Design review of the part shown in the three views and the two pictorial views. Dimensions are in mm from the part's minimum x, y and z. A direction names the side the tool comes from. Round coordinates to 2 decimals unless told otherwise and drop trailing zeros. Order: outer loops, then holes, each group sorted by start corner. A loop starts at its lowest first (then second) coordinate and runs counter-clockwise, first axis right, second up.
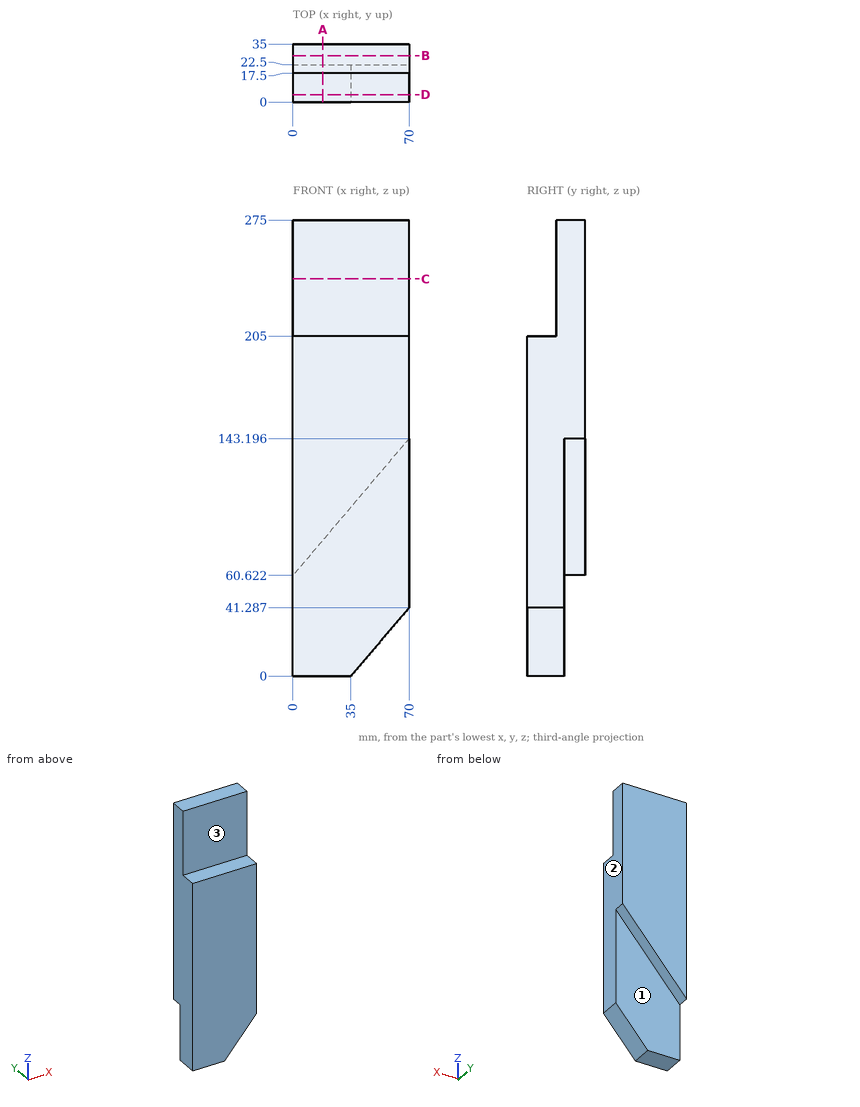
1) To check wall thickness, follow line 1 along Y through (x, z) = (4, 218); line 2 along Y through (x, z) = (9, 61); line 3 along Z through (x, y) = (20, 7). State the ranges of each line that lie inside material, in increasing order.
Results:
line 1: y = 17.5 to 35
line 2: y = 0 to 22.5
line 3: z = 0 to 205
2) Take a section at A-A on x = 18. Give the boundary of the cut face in (y, z) (1 decimal), plus the area to 3 significant figures.
Results:
outline: (0, 0) - (22.5, 0) - (22.5, 81.9) - (35, 81.9) - (35, 275) - (17.5, 275) - (17.5, 205) - (0, 205) - close
area: 7,380 mm2
3) Take a section at C-C on z = 239.5. Give the boundary of the cut face in (x, y), plus the area to 4 significant figures.
Results:
outline: (0, 17.5) - (70, 17.5) - (70, 35) - (0, 35) - close
area: 1,225 mm2
4) Clearance check with flat-ended pins moving along their axes: P1, Ø19, axis at x = 39.5, y = 6, coming from the +Z side; P2, Ø21, axis at x = 17.5, z = 43, coming from the +Y side; P3, Ø4, axis at x = 35, y = 28, coming from the -Z side. State where each tip first meets the part, or that it passes through.
Results:
P1: stops at z = 205
P2: stops at y = 22.5
P3: stops at z = 99.55
5) Take a section at D-D on y = 4.5. Give the boundary of the cut face in (x, z), plus the area to 3 significant figures.
Results:
outline: (0, 0) - (35, 0) - (70, 41.29) - (70, 205) - (0, 205) - close
area: 13,600 mm2
6) Take a section at B-B on y = 28. Give the boundary of the cut face in (x, z).
Results:
outline: (0, 60.62) - (70, 143.2) - (70, 275) - (0, 275) - close
7) For the marked faces 1, 2 and 3, list the 3-axis set-ups (+Z, -Z, +X, -X, +Y, -Y) from which the entire face can be reached by the end or side of a thin tool; tool diameter is ignored.
Results:
face 1: -Z, +X, +Y
face 2: +Z, -Z, +X, +Y, -Y
face 3: +Z, +X, -X, -Y
